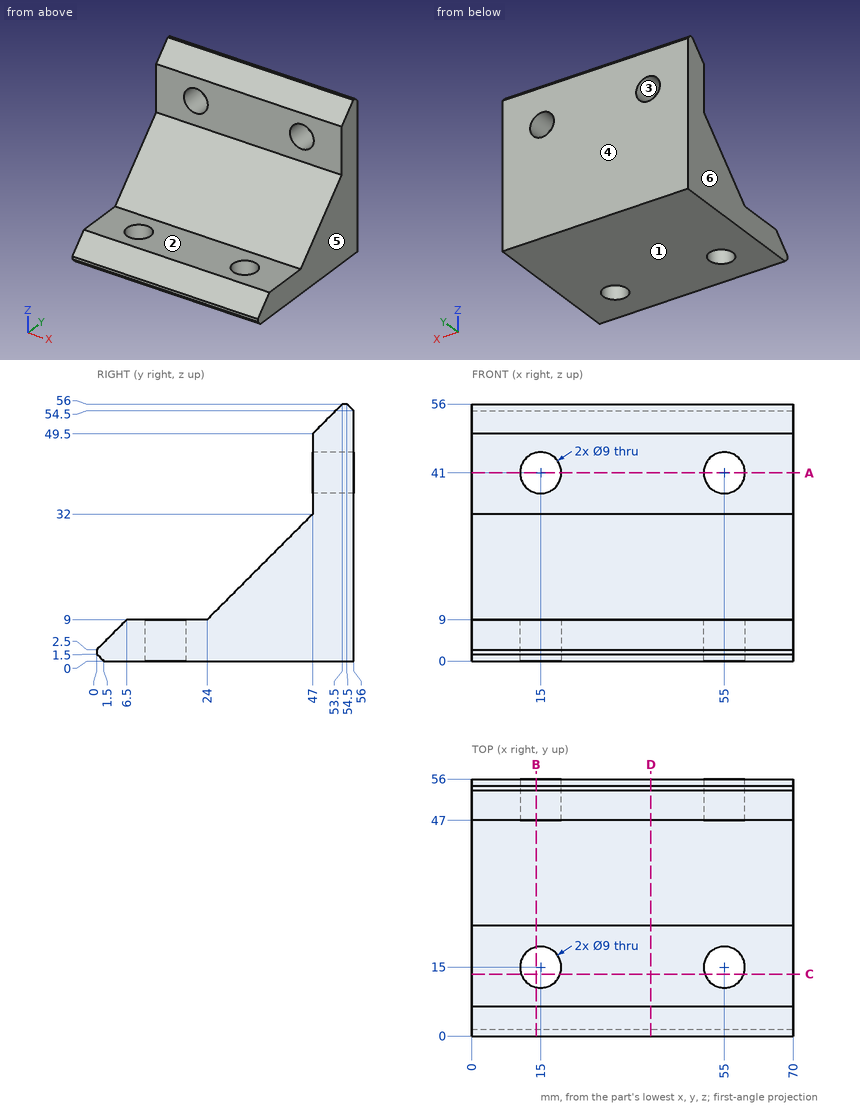
Here's the drawing with two shaded views (mm, measured from the low corner). I have some questions. A direction names the side the tool comes from. Give positions to 0.01 mm unless a question says otherwise; leave off trailing zeros. Write each loop counter-clockwise with the first axis right and the second up, starting at its lowest first coordinate (ties: lowest second). Pieces come first, ordered by that corner, then holes. Notation, with made-up numbers: (-23.75, 82.5) -> (-0.75, 82.5) arc R24 ccw to (-0.75, 109.5) -> close; hole circle Ø8 at (39, 65). An arc over 180 degrees is marked (long way). One line per item, written item: value.
Q1. Which directions (+Z, -Z, +X, -X, +Y, -Y) give clear straight access to the entire face, cutting with the end or side of a thin tool? Please do the marked faces 1 and 2.
Results found:
face 1: -Z, +X, -X, +Y, -Y
face 2: +Z, +X, -X, -Y
Q2. Imagine slicing it at B-B on x = 14. Please give me the cut outline in (y, z).
Results found:
outline: (0, 1.5) -> (1.5, 0) -> (10.61, 0) -> (10.61, 9) -> (6.5, 9) -> (0, 2.5) -> close; (19.39, 0) -> (56, 0) -> (56, 36.61) -> (47, 36.61) -> (47, 32) -> (24, 9) -> (19.39, 9) -> close; (47, 45.39) -> (56, 45.39) -> (56, 54.5) -> (54.5, 56) -> (53.5, 56) -> (47, 49.5) -> close
Q3. Imagine slicing it at D-D on x = 39. Please give me the cut outline in (y, z), and give its area (3 significant figures).
Results found:
outline: (0, 1.5) -> (1.5, 0) -> (56, 0) -> (56, 54.5) -> (54.5, 56) -> (53.5, 56) -> (47, 49.5) -> (47, 32) -> (24, 9) -> (6.5, 9) -> (0, 2.5) -> close
area: 1,150 mm^2
Q4. Imagine slicing it at A-A on z = 41. Please give me the cut outline in (x, y).
Results found:
outline: (0, 47) -> (10.5, 47) -> (10.5, 56) -> (0, 56) -> close; (19.5, 47) -> (50.5, 47) -> (50.5, 56) -> (19.5, 56) -> close; (59.5, 47) -> (70, 47) -> (70, 56) -> (59.5, 56) -> close
Q5. For P1, Ø10.5, axis at x = 15, y = 15, coming from the +Z side; P2, Ø19, axis at x = 17.5, z = 44.5, coming from the -Y side; P3, Ø1.5, axis at x = 51, y = 37, coming from the +Z side, each with a flat end and sliding along its axis, tell me the tip position at first contact or that it passes through.
Results found:
P1: stops at z = 9
P2: stops at y = 47
P3: stops at z = 22.75
Q6. Please list where these lines run through material, in increasing order: line 1 (Z direction, x = 8, y = 17.5); line 2 (Y direction, x = 50.5, z = 53); line 3 (Y direction, x = 65, z = 32.5). Write a range as [from, to].
Results found:
line 1: z = [0, 9]
line 2: y = [50.5, 56]
line 3: y = [47, 56]
Q7. We'd pull the mould along X, two halves only. Please class the marked faces 3, 4, 5 and 6: +X half, -X half, draft (parallel to the pull), parting line (faces both ways), or undercut.
Results found:
face 3: undercut
face 4: draft
face 5: +X half
face 6: -X half
Q8. Imagine slicing it at C-C on y = 13.5. Please give me the cut outline in (x, z).
Results found:
outline: (0, 0) -> (10.76, 0) -> (10.76, 9) -> (0, 9) -> close; (19.24, 0) -> (50.76, 0) -> (50.76, 9) -> (19.24, 9) -> close; (59.24, 0) -> (70, 0) -> (70, 9) -> (59.24, 9) -> close
